Geometry check sheet. Reference: the model listing, model coordinates, mm. A direction names the side the tool comes from. Give positions to 0.01 mm unless a question says otherwise; leave off trailing zeros. Order: outer loops, then holes, each group sorted by start corner. A loop starts at its lowest first (then second) coordinate and runs counter-clockwise, first axis right, second up.
from build123d import *

# Parameters (mm, degrees)
ESQUISSE1_W             = 98
ESQUISSE1_H             = 60
BOSS_EXTRU_1_DEPTH      = 1.6
ESQUISSE2_R             = 1.6
ENL_V_MAT_EXTRU_1_DEPTH = 58.476603936
ESQUISSE3_W             = 97.9
ESQUISSE3_H             = 39
BOSS_EXTRU_2_DEPTH      = 11.05
ESQUISSE4_W             = 76.3
ESQUISSE4_H             = 25
ENL_V_MAT_EXTRU_2_DEPTH = 0.5
ESQUISSE5_W             = 40
ESQUISSE5_H             = 3
BOSS_EXTRU_3_DEPTH      = 2


with BuildPart() as part:
    # Esquisse1 → Boss.-Extru.1 (new body)
    with BuildSketch(Plane.XY):
        Rectangle(ESQUISSE1_W, ESQUISSE1_H)
    extrude(amount=BOSS_EXTRU_1_DEPTH)

    # Esquisse2 → Enlèv. mat.-Extru.1 (cut, through all)
    with BuildSketch(Plane.XY.offset(1.6)):
        with Locations((-46.5, 27.5)):
            Circle(ESQUISSE2_R)
        with Locations((-46.5, -27.5)):
            Circle(ESQUISSE2_R)
        with Locations((46.5, -27.5)):
            Circle(ESQUISSE2_R)
        with Locations((46.5, 27.5)):
            Circle(ESQUISSE2_R)
    extrude(amount=-ENL_V_MAT_EXTRU_1_DEPTH, mode=Mode.SUBTRACT)

    # Esquisse3 → Boss.-Extru.2 (add)
    with BuildSketch(Plane.XY.offset(1.6)):
        Rectangle(ESQUISSE3_W, ESQUISSE3_H)
    extrude(amount=BOSS_EXTRU_2_DEPTH)

    # Esquisse4 → Enlèv. mat.-Extru.2 (cut)
    with BuildSketch(Plane.XY.offset(12.65)):
        Rectangle(ESQUISSE4_W, ESQUISSE4_H)
    extrude(amount=-ENL_V_MAT_EXTRU_2_DEPTH, mode=Mode.SUBTRACT)

    # Esquisse5 → Boss.-Extru.3 (add)
    with BuildSketch(Plane.XY.offset(1.6)):
        with Locations((-19, 28.4)):
            Rectangle(ESQUISSE5_W, ESQUISSE5_H)
    extrude(amount=BOSS_EXTRU_3_DEPTH)


solid = part.part
Item 1: Sectioned sample at A-A (y = -27.5). Enter the section's corners in (x, z).
Reported:
outline: (-49, 0) - (-48.1, 0) - (-48.1, 1.6) - (-49, 1.6) - close; (-44.9, 0) - (44.9, 0) - (44.9, 1.6) - (-44.9, 1.6) - close; (48.1, 0) - (49, 0) - (49, 1.6) - (48.1, 1.6) - close
Item 2: Sectioned sample at B-B (x = 46.5). Enter the section's corners in (y, z), and give its area (3 significant figures).
Reported:
outline: (-30, 0) - (-29.1, 0) - (-29.1, 1.6) - (-30, 1.6) - close; (-25.9, 0) - (25.9, 0) - (25.9, 1.6) - (19.5, 1.6) - (19.5, 12.65) - (-19.5, 12.65) - (-19.5, 1.6) - (-25.9, 1.6) - close; (29.1, 0) - (30, 0) - (30, 1.6) - (29.1, 1.6) - close
area: 517 mm2
Item 3: Gauge pin test, flat ends, axial feed: pin 1 (1.9 mm diameter, centred on x = 46.5, y = 27.5, fed in from -Z); pin 2 (0.6 mm diameter, centred on y = -2.5, z = 12.5, fed in from -X); pin 3 (5.5 mm diameter, centred on y = -6.5, z = 9, fed in from +X); pin 4 (1.6 mm diameter, centred on y = 28.5, z = 3, fed in from -X). Record the tip position at first contact, or that the pin passes through.
Reported:
pin 1: passes through
pin 2: stops at x = -48.95
pin 3: stops at x = 48.95
pin 4: stops at x = -39
Item 4: Draft check along Y on faces 6 (the flat face through (-1, 0, 0)), 7 (the flat face through (-1, -19.5, 7)), 8 (the cylindrical face through (46.292, 29.086, 0.811)). Enter one of: released by +Y, released by -Y, zero draft, split by the parting line, or undercut.
Reported:
face 6: zero draft
face 7: released by -Y
face 8: undercut
Item 5: Set-up check for faces 1 (the flat face through (-19, 28, 3.6)), 2 (the flat face through (1, 28, 3)), 3 (the flat face through (-19, 26.9, 3)), 4 (the flat face through (-39, 28, 3)), 5 (the flat face through (-1, 0, 12.15)): record each of +Z, -Z, +X, -X, +Y, -Y from which the full face is reachable in a straight line by a thin tool's end or side.
Reported:
face 1: +Z, +X, -X, +Y
face 2: +Z, +X, +Y
face 3: +Z, +X, -X
face 4: +Z, -X, +Y
face 5: +Z
Item 6: Sectioned sample at C-C (y = 6). Enter the section's corners in (x, z).
Reported:
outline: (-49, 0) - (49, 0) - (49, 1.6) - (48.95, 1.6) - (48.95, 12.65) - (38.15, 12.65) - (38.15, 12.15) - (-38.15, 12.15) - (-38.15, 12.65) - (-48.95, 12.65) - (-48.95, 1.6) - (-49, 1.6) - close
Item 7: Scan lines: L1, parallel to Y at x = 46.5, z = 1; L2, parallel to Y at x = -37, z = 2.25; L3, parallel to Z at x = 35.5, y = 22. Record each from-to range of solid material in increasing order.
Reported:
L1: y = -30 to -29.1, -25.9 to 25.9, 29.1 to 30
L2: y = -19.5 to 19.5, 26.9 to 29.9
L3: z = 0 to 1.6
Item 8: Sectioned sample at D-D (x = 28.5). Enter the section's corners in (y, z).
Reported:
outline: (-30, 0) - (30, 0) - (30, 1.6) - (19.5, 1.6) - (19.5, 12.65) - (12.5, 12.65) - (12.5, 12.15) - (-12.5, 12.15) - (-12.5, 12.65) - (-19.5, 12.65) - (-19.5, 1.6) - (-30, 1.6) - close
